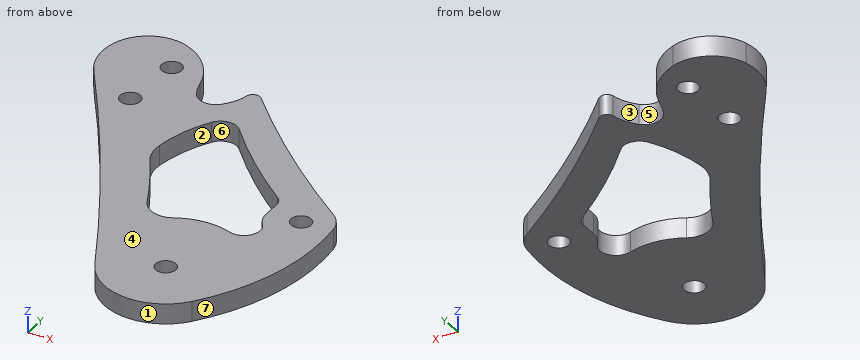
from build123d import *

# Parameters (mm, degrees)
ESQUISSE1_R        = 1.5
ESQUISSE1_R_2      = 1.50110642
BOSS_EXTRU_1_DEPTH = 3


with BuildPart() as part:
    # Esquisse1 → Boss.-Extru.1 (new body)
    with BuildSketch(Plane.XY):
        with BuildLine():
            ThreePointArc((60.026944648, 49.921558504), (72.778337749, 29.898863696), (84.195273994, 9.086369847))
            ThreePointArc((84.195273994, 9.086369847), (91.451273571, 4.140927091), (99.509067829, 7.630753106))
            ThreePointArc((99.509067829, 7.630753106), (105.251720368, 19.156706799), (106.145904128, 32.002955361))
            ThreePointArc((106.145904128, 32.002955361), (105.517176975, 33.787686969), (104.210334733, 35.15616353))
            ThreePointArc((104.210334733, 35.15616353), (92.58899703, 44.531440422), (81.889188019, 54.946112475))
            ThreePointArc((81.889188019, 54.946112475), (80.829609942, 55.239205413), (80.085451585, 54.429985101))
            ThreePointArc((80.085451585, 54.429985101), (79.43974416, 52.594599516), (78.30149473, 51.016636729))
            ThreePointArc((78.30149473, 51.016636729), (76.19777745, 50.272546762), (74.337717048, 51.505215238))
            ThreePointArc((74.337717048, 51.505215238), (73.781586954, 52.671085372), (73.412965229, 53.909088553))
            ThreePointArc((73.412965229, 53.909088553), (71.258227235, 58.277263879), (67.291581582, 61.103847288))
            ThreePointArc((67.291581582, 61.103847288), (62.173852637, 60.880940246), (58.891944342, 56.947758957))
            ThreePointArc((58.891944342, 56.947758957), (58.674610839, 53.307878055), (60.026944648, 49.921558504))
        make_face()
        with Locations((68.285467108, 55.560427953)):
            Circle(ESQUISSE1_R, mode=Mode.SUBTRACT)
        with Locations((101.682075096, 31.433543054)):
            Circle(ESQUISSE1_R, mode=Mode.SUBTRACT)
        with Locations((92.312371453, 13.200094295)):
            Circle(ESQUISSE1_R, mode=Mode.SUBTRACT)
        with Locations((67.535467108, 46.360427953)):
            Circle(ESQUISSE1_R_2, mode=Mode.SUBTRACT)
        with BuildLine():
            Line((96.849719723, 30.848999233), (96.849719723, 33.474650871))
            ThreePointArc((96.849719723, 33.474650871), (96.647309876, 34.343108764), (96.081794601, 35.032587793))
            ThreePointArc((96.081794601, 35.032587793), (89.436975045, 40.671042336), (83.372922141, 46.929880801))
            ThreePointArc((83.372922141, 46.929880801), (81.323140328, 47.752609653), (79.445810973, 46.588941858))
            ThreePointArc((79.445810973, 46.588941858), (77.571604785, 42.607109512), (76.591708968, 38.316720036))
            ThreePointArc((76.591708968, 38.316720036), (76.69683067, 36.288635677), (77.467153905, 34.409598995))
            ThreePointArc((77.467153905, 34.409598995), (79.992055499, 30.078906011), (82.254048976, 25.605270433))
            ThreePointArc((82.254048976, 25.605270433), (84.350090923, 23.753861276), (87.134236378, 24.017758597))
            ThreePointArc((87.134236378, 24.017758597), (91.023623533, 25.188476532), (95.051173024, 24.662398573))
            ThreePointArc((95.051173024, 24.662398573), (97.816197879, 25.543673578), (97.709238653, 28.443771474))
            ThreePointArc((97.709238653, 28.443771474), (97.07105369, 29.571903567), (96.849719723, 30.848999233))
        make_face(mode=Mode.SUBTRACT)
    extrude(amount=BOSS_EXTRU_1_DEPTH)


solid = part.part
Geometry check sheet. Reference: the model listing, model coordinates, mm. Face numbers are marked on the shaded views. A direction names the side the tool comes from. Give positions to 0.01 mm unless a question says otherwise; leave off trailing zeros. Order: outer loops, then holes, each group sorted by start corner. A loop starts at its lowest first (then second) coordinate and runs counter-clockwise, first axis right, second up.
1) Draft check along Y on the marked faces 4, 5, 6 and 7. Enter one of: released by +Y, released by -Y, zero draft, split by the parting line, or undercut.
Results are:
face 4: zero draft
face 5: released by +Y
face 6: undercut
face 7: split by the parting line
2) Material ranges on probe 1 along X at (y, z) = (54.5, 2); probe 2 along X at (y, z) = (45, 2); probe 3 along Y at (x, z) = (68, 2.2), recorded low to high.
Results are:
probe 1: x = 58.57 to 67.22, 69.35 to 73.27, 80.1 to 82.31
probe 2: x = 63.33 to 66.9, 68.17 to 78.57, 85.12 to 92.06
probe 3: y = 37.74 to 44.93, 47.79 to 54.09, 57.03 to 60.79
3) Cross-section at A-A (x = 85). Record the boundary of the cut face in (y, z).
Results are:
outline: (7.78, 0) - (23.61, 0) - (23.61, 3) - (7.78, 3) - close; (45.13, 0) - (51.71, 0) - (51.71, 3) - (45.13, 3) - close
4) Cross-section at B-B (y = 42). Record the boundary of the cut face in (x, z), then the cut area to 3 significant figures.
Results are:
outline: (65.29, 0) - (77.37, 0) - (77.37, 3) - (65.29, 3) - close; (88.05, 0) - (95.51, 0) - (95.51, 3) - (88.05, 3) - close
area: 58.6 mm2
5) Cross-section at D-D (y = 21). Record the boundary of the cut face in (x, z).
Results are:
outline: (77.88, 0) - (105.7, 0) - (105.7, 3) - (77.88, 3) - close
6) Cross-section at C-C (z = 0.65). Record the boundary of the cut face in (x, y), then the cut area to 3 significant figures.
Results are:
outline: (58.89, 56.95) arc R8.36 ccw to (60.03, 49.92) arc R363.4 cw to (84.2, 9.09) arc R9.1 ccw to (99.51, 7.63) arc R33 ccw to (106.15, 32) arc R4.5 ccw to (104.21, 35.16) arc R160.5 cw to (81.89, 54.95) arc R1.05 ccw to (80.09, 54.43) arc R6.81 cw to (78.3, 51.02) arc R2.5 cw to (74.34, 51.51) arc R8.31 cw to (73.41, 53.91) arc R9.97 ccw to (67.29, 61.1) arc R6.34 ccw to start; hole circle Ø3 at (67.54, 46.36); hole circle Ø3 at (68.29, 55.56); hole (76.59, 38.32) arc R6.05 ccw to (77.47, 34.41) arc R83.98 cw to (82.25, 25.61) arc R3.52 ccw to (87.13, 24.02) arc R9.69 cw to (95.05, 24.66) arc R2.4 ccw to (97.71, 28.44) arc R3.8 cw to (96.85, 30.85) - (96.85, 33.47) arc R1.96 ccw to (96.08, 35.03) arc R89.37 cw to (83.37, 46.93) arc R2.45 ccw to (79.45, 46.59) arc R20.47 ccw to start; hole circle Ø3 at (92.31, 13.2); hole circle Ø3 at (101.68, 31.43)
area: 1,050 mm2
7) Gauge pin test, flat end, axial feed: pin 1 (2.5 mm diameter, centred on x = 67.54, y = 46.36, fed in from -Z). Record the tip position at first contact, or that the pin passes through.
Results are:
pin 1: passes through
8) Tool access check on the marked faces 1, 2 and 3. Record the directions out of +Z, -Z, +X, -X, +Y, -Y that give a thin tool (end or side, any length) a straight path to the whole face; none if there is none.
Results are:
face 1: +Z, -Z, -Y
face 2: +Z, -Z
face 3: +Z, -Z, +Y
